from build123d import *

# Parameters (mm, degrees)
SHELL2_T = -0.0254


with BuildPart() as part:
    # Sweep2: sweep along a path in Sketch2
    with BuildLine(Plane(origin=(0, 0, 0), x_dir=(0, 0, -1), z_dir=(1, 0, 0))) as sweep2_path:
        Line((-325, 0), (-502.8, -149.191914423))
    # Sketch3 → Sweep2 (sweep)
    with BuildSketch(Plane.XY.offset(325)):
        Polygon((200, 0), (-200, 0), (-275, -500), (-175, -600), (175, -600), (275, -500), align=None)
    sweep(path=sweep2_path.line)

    # Shell2
    shell2_openings = [part.faces().sort_by_distance(p)[0] for p in [
        (0, -457.451501444, 502.8),
    ]]
    offset(amount=SHELL2_T, openings=shell2_openings, kind=Kind.INTERSECTION)


solid = part.part
CAD build for the part. Positions are in the model's coordinates, mm. Coordinates: 2 decimals unless noted, no trailing zeros. Write each loop counter-clockwise with the first axis right and the second up, starting at its lowest first coordinate (ties: lowest second). Pieces come first, ordered by that corner, then holes. Notation, with made-up numbers: M 25,21.5 L 38,21.5 A16 cw 38,45.5 Z; hole C 33,34 d10. An arc over 180 degrees is marked long. Answer as a JSON object with one key per item and string values. Group by question number.
1) Pin check, flat tips, straight feed: pin 1 Ø4 at (x, z) = (40, 375.5) entering from +Y; pin 2 Ø5 at (x, z) = (73, 464) entering from -Y; pin 3 Ø4 at (x, z) = (-170.5, 398) entering from -Y. Stop position of each tip, or through.
2) Saw through at C-C (z = 418). Write the cut outline in (x, y).
3) Saw through at B-B (y = -73). Write the cut outline in (x, z), plus the area to 3 significant figures.
Values follow:
{
 "1": {"pin 1": "stops at y = -40.7", "pin 2": "stops at y = -718.73", "pin 3": "stops at y = -662.93"},
 "2": {"outline": "M -275,-578.04 L -175,-678.04 L 175,-678.04 L 275,-578.04 L 200,-78.04 L -200,-78.04 Z; hole M -274.97,-578.02 L -174.99,-678 L 174.99,-678 L 274.97,-578.02 L 199.98,-78.07 L -199.98,-78.07 Z"},
 "3": {"outline": "M -210.95,325 L 210.95,325 L 200,412 L -200,412 Z; hole M -210.92,325.03 L 210.92,325.03 L 199.98,411.96 L -199.98,411.96 Z", "area": "31.0 mm2"}
}
